from build123d import *

# Parameters (mm, degrees)
F0_R            = 85.725
F0_R_2          = 63.5
F1_DEPTH        = 203.2
F3_DEPTH        = 9.525
F3_COPIES_COUNT = 4


# Not quite as in the source:
# - after a boolean that leaves OpenCascade's solid faulty, fix() repairs it
# - a pattern or mirror of a feature is missing from the dataset's text; its kind, count and spacing are read off the source's solid


with BuildPart() as f1:
    # F0 (on Top) → F1 (new body)
    with BuildSketch(Plane.XY):
        Circle(F0_R)
        Circle(F0_R_2, mode=Mode.SUBTRACT)
    extrude(amount=F1_DEPTH)

    # F2 (on face) → F3 (join)
    with BuildSketch(Plane(origin=(0, 0, 0), x_dir=(1, 0, 0), z_dir=(0, 0, -1))):
        with BuildLine():
            Line((-7.874, 85.3626132976), (-7.874, 77.7426132976))
            Line((-7.874, 77.7426132976), (7.874, 77.7426132976))
            Line((7.874, 77.7426132976), (7.874, 85.3626132976))
            ThreePointArc((7.874, 85.3626132976), (0, 85.725), (-7.874, 85.3626132976))
        make_face()
    f3 = extrude(amount=F3_DEPTH)

    # F3_copies: F3 ×4 about axis
    f3_copies_axis = Axis((0, 0, 0), (0, 0, 1))
    for i in range(1, F3_COPIES_COUNT):
        add(f3.rotate(f3_copies_axis, i * 360 / F3_COPIES_COUNT))

    add(f1.part.fix(), mode=Mode.REPLACE)


solid = f1.part
Source: CAD feature listing. Evaluate the final solid. Frame: model axes, mm. A direction names the side the tool comes from. Coordinates: 2 decimals unless noted, no trailing zeros. Loops run counter-clockwise (first coordinate to the right, second up) from the corner with the lowest first, then second, coordinate; pieces in that order, holes last. Notation, with made-up numbers: (0.5, -1.75) - (5.5, -1.75) arc R7 ccw to (5.5, 7.25) - close; hole circle Ø10 at (3, 85). An arc over 180 degrees is marked (long way). One line per item, written item: value. Start each with the question number.
1. Section C-C (z = 184.5). Return the cut outline in (x, y) (3 decimals).
2. Mould query, pull axis X, two halves, no side actions, for faces 1 (the flat face through (7.874, -81, -5)), 2 (the flat face through (77.743, 0, -5)), 3 (the flat face through (82, -7.874, -5)). Classes: pulls with the +X half, pulls with the -X half, needs draft (parallel to the pull), parting line crosses it, or undercut.
3. Section A-A (y = 0). Return the cut outline in (x, z) (3 decimals), and give its area (3 significant figures).
4. Section D-D (y = 53.5). Return the cut outline in (x, z).
5. Ray query, L1, parallel to Y at x = 0, z = 111.5 (3 decimals); L2, parallel to Z at x = 70, y = -47.5; L3, parallel to Y at x = 4.5, z = 46.5. Return the intervals inside material, ascending.
6. Set-up query: faces 4 (the flat face through (-7.874, 81, -5)), 5 (the flat face through (7.874, 82, -5)), 6 (the flat face through (-81, -7.874, -5)), 7 (the flat face through (81, 7.874, -5)), 8 (the flat face through (0, -77.743, -5)). Return all of +Z, -Z, +X, -X, +Y, -Y with unobstructed straight access to the full face (end or side cutting, diameter ignored); none if empty.
7. Contact query for flat-ended pins moving along their axis: P1, Ø3, axis at x = -55.5, z = 14, coming from the +Y side; P2, Ø6, axis at y = -81, z = -6, coming from the -X side; P3, Ø8, axis at x = 41, z = 103, coming from the -Y side. Output: stop coordinate, or through.
Verdict:
1. outline: circle Ø171.45 at (0, 0); hole circle Ø127 at (0, 0)
2. face 1: pulls with the +X half
2. face 2: undercut
2. face 3: needs draft
3. outline: (-85.725, -9.525) - (-77.743, -9.525) - (-77.743, 0) - (-63.5, 0) - (-63.5, 203.2) - (-85.725, 203.2) - close; (63.5, 0) - (77.743, 0) - (77.743, -9.525) - (85.725, -9.525) - (85.725, 203.2) - (63.5, 203.2) - close
3. area: 9,180 mm2
4. outline: (-66.98, 0) - (-34.21, 0) - (-34.21, 203.2) - (-66.98, 203.2) - close; (34.21, 0) - (66.98, 0) - (66.98, 203.2) - (34.21, 203.2) - close
5. L1: y = -85.725 to -63.5, 63.5 to 85.725
5. L2: z = 0 to 203.2
5. L3: y = -85.61 to -63.34, 63.34 to 85.61
6. face 4: -Z, -X, +Y, -Y
6. face 5: -Z, +X, +Y, -Y
6. face 6: -Z, +X, -X, -Y
6. face 7: -Z, +X, -X, +Y
6. face 8: -Z, +X, -X
7. P1: stops at y = 66.58
7. P2: stops at x = -7.87
7. P3: stops at y = -77.33
